Autodesk Inventor part; units mm, degrees
ref_plane "YZ Plane" through (0, 0, 0) normal (1, 0, 0) x (0, 1, 0)
ref_plane "XZ Plane" through (0, 0, 0) normal (0, 1, 0) x (-1, 0, 0)
ref_plane "XY Plane" through (0, 0, 0) normal (0, 0, 1) x (1, 0, 0)
sketch "Sketch1" plane through (0, 0, 0) normal (1, 0, 0) x (0, 1, 0)
  line L0 (12, -9) -> (2, -9)
  line L1 (2, -9) -> (2, 41)
  line L2 (2, 41) -> (7, 41)
  line L3 (7, 41) -> (7, 31)
  line L4 (7, 31) -> (12, 31)
  line L5 (12, 31) -> (12, -9)
  line L6 (2, 111) -> (12, 111)
  line L7 (12, 111) -> (12, 71)
  line L8 (12, 71) -> (7, 71)
  line L9 (7, 71) -> (7, 61)
  line L10 (7, 61) -> (2, 61)
  line L11 (2, 61) -> (2, 111)
  line L12 (7, 54.5) -> (7, 55)
  line L13 (7, 55) -> (62, 55)
  arc A0 (64, 57) -> (62, 55) centre (64, 55) ccw
  line L14 (64, 57) -> (65, 57)
  arc A1 (67, 55) -> (65, 57) centre (65, 55) ccw
  line L15 (67, 55) -> (102, 55)
  arc A2 (104, 57) -> (102, 55) centre (104, 55) ccw
  line L16 (104, 57) -> (105, 57)
  arc A3 (107, 55) -> (105, 57) centre (105, 55) ccw
  line L17 (107, 55) -> (107, 47)
  arc A4 (105, 45) -> (107, 47) centre (105, 47) ccw
  line L18 (105, 45) -> (104, 45)
  arc A5 (102, 47) -> (104, 45) centre (104, 47) ccw
  line L19 (102, 47) -> (67, 47)
  arc A6 (65, 45) -> (67, 47) centre (65, 47) ccw
  line L20 (65, 45) -> (64, 45)
  arc A7 (62, 47) -> (64, 45) centre (64, 47) ccw
  line L21 (62, 47) -> (7, 47)
  line L22 (7, 47) -> (7, 47.5)
  line L23 (7, 47.5) -> (-5, 47.5)
  line L24 (-5, 47.5) -> (-5, 41)
  line L25 (-5, 41) -> (0, 41)
  line L26 (0, 41) -> (0, 2.0396)
  line L27 (0, 2.0396) -> (0.3922, 1.9612)
  line L28 (0.3922, 1.9612) -> (0, 1.0198)
  line L29 (0, 1.0198) -> (0, 0)
  line L30 (0, 0) -> (-0.3922, 0.0784)
  line L31 (-0.3922, 0.0784) -> (-15.377, -35.885)
  line L32 (-15.377, -35.885) -> (-19.9924, -33.9619)
  line L33 (-19.9924, -33.9619) -> (-22.4924, -39.9619)
  line L34 (-22.4924, -39.9619) -> (-11.4155, -44.5773)
  line L35 (-11.4155, -44.5773) -> (-11.2232, -44.1158)
  line L36 (-11.2232, -44.1158) -> (39.5461, -65.2696)
  arc A8 (42.1615, -64.1927) -> (39.5461, -65.2696) centre (41.3922, -66.0388) ccw
  line L37 (42.1615, -64.1927) -> (43.0845, -64.5773)
  arc A9 (44.1615, -67.1927) -> (43.0845, -64.5773) centre (42.3153, -66.4235) ccw
  line L38 (44.1615, -67.1927) -> (76.4692, -80.6542)
  arc A10 (79.0845, -79.5773) -> (76.4692, -80.6542) centre (78.3153, -81.4235) ccw
  line L39 (79.0845, -79.5773) -> (80.0076, -79.9619)
  arc A11 (81.0845, -82.5773) -> (80.0076, -79.9619) centre (79.2384, -81.8081) ccw
  line L40 (81.0845, -82.5773) -> (78.0076, -89.9619)
  arc A12 (75.3922, -91.0388) -> (78.0076, -89.9619) centre (76.1615, -89.1927) ccw
  line L41 (75.3922, -91.0388) -> (74.4692, -90.6542)
  arc A13 (73.3922, -88.0388) -> (74.4692, -90.6542) centre (75.2384, -88.8081) ccw
  line L42 (73.3922, -88.0388) -> (41.0845, -74.5773)
  arc A14 (38.4692, -75.6542) -> (41.0845, -74.5773) centre (39.2384, -73.8081) ccw
  line L43 (38.4692, -75.6542) -> (37.5461, -75.2696)
  arc A15 (36.4692, -72.6542) -> (37.5461, -75.2696) centre (38.3153, -73.4235) ccw
  line L44 (36.4692, -72.6542) -> (-14.3001, -51.5004)
  line L45 (-14.3001, -51.5004) -> (-14.1078, -51.0388)
  line L46 (-14.1078, -51.0388) -> (-25.1847, -46.4235)
  line L47 (-25.1847, -46.4235) -> (-27.6847, -52.4235)
  line L48 (-27.6847, -52.4235) -> (-23.0693, -54.3465)
  line L49 (-23.0693, -54.3465) -> (-38.8385, -92.1927)
  line L50 (-38.8385, -92.1927) -> (-47.3001, -86.5004)
  line L51 (-47.3001, -86.5004) -> (-30.377, -45.885)
  line L52 (-30.377, -45.885) -> (-39.6078, -42.0388)
  line L53 (-39.6078, -42.0388) -> (-35.7616, -32.8081)
  line L54 (-35.7616, -32.8081) -> (-26.5308, -36.6542)
  line L55 (-26.5308, -36.6542) -> (-10, 3.0198)
  line L56 (-10, 3.0198) -> (-10, 46)
  line L57 (-10, 46) -> (-20, 46)
  line L58 (-20, 46) -> (-20, 56)
  line L59 (-20, 56) -> (-10, 56)
  line L60 (-10, 56) -> (-10, 100)
  line L61 (-10, 100) -> (0, 102)
  line L62 (0, 102) -> (0, 61)
  line L63 (0, 61) -> (-5, 61)
  line L64 (-5, 61) -> (-5, 54.5)
  line L65 (-5, 54.5) -> (7, 54.5)
  line L66 (0, 51) -> (107, 51)
  line L67 (79.5461, -86.2696) -> (-37.6847, -37.4235)
sketch "Sketch2" plane through (0, 0, 0) normal (1, 0, 0) x (0, 1, 0)
  line L0 (0, 0) -> (0, 51)
  line L1 (0, 51) -> (15, 51)
  line L2 (15, 51) -> (15, 101)
  line L3 (15, 101) -> (65, 101)
  line L4 (101.707, 46.9392) -> (84.707, 46.9392)
  line L5 (84.707, 46.9392) -> (34.707, 46.9392)
  line L6 (15, 51) -> (15, 60)
  line L7 (0, 0) -> (0, 1)
  line L8 (0, 1) -> (110.5886, -21.1178)
  line L9 (50.3822, 41.5) -> (30.3822, 41.5)
  line L10 (30.3822, 41.5) -> (30.3822, 0.5)
  line L11 (30.3822, 0.5) -> (50.3822, 0.5)
  line L12 (50.3822, 0.5) -> (50.3822, 41.5)
  line L13 (50.3822, 0.5) -> (45.3822, 0.5)
  line L14 (45.3822, 0.5) -> (45.3822, -3.5)
  line L15 (45.3822, -3.5) -> (35.3822, -3.5)
  circle A0 centre (45.3822, -3.5) radius 2
  circle A1 centre (35.3822, -3.5) radius 2
  line L16 (50.3822, 21) -> (30.3822, 21)
  circle A2 centre (45.3822, 45.5) radius 2
  circle A3 centre (35.3822, 45.5) radius 2
  line L17 (65, 101) -> (65, -12.0001)
  line L18 (0, 51) -> (107.1279, 51)
  line L19 (65, 51) -> (55, 51)
  line L20 (15, 51) -> (25, 51)
  line L21 (-5.3847, -50.9231) -> (-24.6156, -97.0769)
  line L22 (-24.6156, -97.0769) -> (21.5382, -116.3077)
  line L23 (21.5382, -116.3077) -> (65, -12.0001)
  line L24 (15, 51) -> (15, -19)
  line L25 (-5.3847, -50.9231) -> (7.9166, -19)
  line L26 (15, -19) -> (7.9166, -19)
  line L27 (30.9296, -55.7624) -> (12.468, -48.0701)
  line L28 (12.468, -48.0701) -> (28.2374, -10.224)
  line L29 (28.2374, -10.224) -> (46.6989, -17.9163)
  line L30 (46.6989, -17.9163) -> (30.9296, -55.7624)
  circle A4 centre (43.622, -12.3009) radius 2
  circle A5 centre (34.3912, -8.4548) radius 2
  circle A6 centre (24.7757, -57.5317) radius 2
  circle A7 centre (15.545, -53.6855) radius 2
  line L31 (65, 51) -> (65, 41)
  line L32 (65, 41) -> (63.5, 41)
  line L33 (63.5, 41) -> (63.5, 61)
  line L34 (63.5, 61) -> (65, 61)
  line L35 (65, 61) -> (65, 41)
  line L36 (63.5, 61) -> (57.5, 61)
  line L37 (57.5, 61) -> (56, 61)
  line L38 (56, 61) -> (56, 41)
  line L39 (56, 41) -> (57.5, 41)
  line L40 (57.5, 41) -> (57.5, 61)
  line L41 (65, 51) -> (60.5, 51)
  circle A8 centre (60.5, 51) radius 1.5
  line L42 (44.6152, -60.9232) -> (43.2306, -60.3463)
  line L43 (43.2306, -60.3463) -> (35.5383, -78.8078)
  line L44 (35.5383, -78.8078) -> (36.9229, -79.3847)
  line L45 (29.9998, -76.5001) -> (28.6152, -75.9231)
  line L46 (28.6152, -75.9231) -> (36.3076, -57.4616)
  line L47 (36.3076, -57.4616) -> (37.6922, -58.0386)
  line L48 (37.6922, -58.0386) -> (29.9998, -76.5001)
  circle A9 centre (36.6152, -68.4232) radius 1.5
  line L49 (-1.5387, -106.6923) -> (40, -7)
  line L50 (40, 101) -> (40, -7)
  line L51 (40, -68.0997) -> (40, -71.9997)
  circle A10 centre (-1.2309, -52.6538) radius 1.5
  line L52 (5.3845, -44.5769) -> (-2.3078, -63.0385)
  line L53 (-0.9232, -63.6154) -> (6.7691, -45.1539)
  line L54 (6.7691, -45.1539) -> (5.3845, -44.5769)
  line L55 (-2.3078, -63.0385) -> (-0.9232, -63.6154)
  line L56 (-0.1539, -42.2692) -> (-7.8463, -60.7308)
  line L57 (-7.8463, -60.7308) -> (-9.2309, -60.1538)
  line L58 (-1.5386, -41.6923) -> (-0.1539, -42.2692)
  line L59 (15, 41) -> (16.5, 41)
  line L60 (16.5, 41) -> (16.5, 61)
  line L61 (16.5, 61) -> (15, 61)
  line L62 (22.5, 61) -> (24, 61)
  line L63 (24, 61) -> (24, 41)
  line L64 (24, 41) -> (22.5, 41)
  line L65 (22.5, 41) -> (22.5, 61)
  circle A11 centre (19.5, 51) radius 1.5
  dimension "d0" = 51
  dimension "d1" = 15
  dimension "d2" = 50
  dimension "d3" = 50
  dimension "d11" = 17
  dimension "d12" = 50
  dimension "d23" = 9
  dimension "d34" = 1
  dimension "d35" = 78.69
  dimension "d36" = 20
  dimension "d37" = 41
  dimension "d38" = 5
  dimension "d39" = 4
  dimension "d40" = 10
  dimension "d41" = 4
  dimension "d42" = 4
  dimension "d43" = 10
  dimension "d47" = 10
  dimension "d48" = 70
  dimension "d86" = 10
  dimension "d87" = 1.5
  dimension "d88" = 20
  dimension "d89" = 6
  dimension "d90" = 1.5
  dimension "d91" = 20
  dimension "d92" = 4.5
  dimension "d93" = 3
extrude "Extrusion1" add sketch "Sketch2" along normal blind 1.5 contours L24 L59 L60 L18 A11 L65 L64 L63 L50 L9 L10 L11 L8 | L8 L49 L29 L28 L27 L22 L21 L57 L56 L58 L25 L26 L24 | L2 L61 L60 L18 | L18 L60 L59 L24 | L50 L15 A0 L14 L11 L12 L9 L5 A2 L38 L39 L40 L33 L32 L17 L8 | L8 L23 L42 L43 L44 L22 L49 L27 L30 L29 | L60 L61 L2 L3 L50 L18 L63 L62 L65 A11 | L50 L11 L14 A0 L15 | A11 L18 | L18 A11 | L32 L33 L5 L17 | L23 L51 L43 L42 | L58 L56 L57 L21 L25 | L5 L33 L18 L17 | L23 L44 L43 L51 | L3 L17 L34 L36 L37 L38 L18 L50 | L65 L62 L63 L18 | L18 L63 L64 L65 | L5 L40 L18 A8 L33 | L18 L33 L34 L17 | L18 L38 L5 A2 L50 | L40 L39 L38 L5 | L5 L38 L18 L40 | L18 A8 L40 L36 L33 | L18 L38 L37 L40 | A8 L18 | L18 A8 | L45 L46 L47 L48 | A9 | A10 | L54 L53 L55 L52
sketch "Sketch3" plane through (1.5, 0, 0) normal (1, 0, 0) x (0, 0, -1)
  line L0 (-101, 65) -> (-101, 15)
  line L1 (-101, 65) -> (-101, 55)
  line L2 (-101, 55) -> (-106, 55)
  line L3 (-106, 55) -> (-106, 35)
  line L4 (-106, 35) -> (-101, 35)
  line L5 (-101, 55) -> (-101, 50)
  line L6 (-101, 50) -> (-102.5, 50)
  line L7 (-102.5, 50) -> (-102.5, 40)
  line L8 (-102.5, 40) -> (-101, 40)
  line L9 (-101, 40) -> (-101, 50)
  line L10 (-1, 0) -> (21.1178, 110.5886)
  line L11 (116.3077, 21.5382) -> (97.0769, -24.6156)
  line L12 (112.4616, 12.3074) -> (117.0769, 10.3843)
  line L13 (117.0769, 10.3843) -> (109.3846, -8.0772)
  line L14 (109.3846, -8.0772) -> (104.7692, -6.1541)
  line L15 (110.5385, 7.692) -> (111.9231, 7.1151)
  line L16 (111.9231, 7.1151) -> (108.0769, -2.1156)
  line L17 (108.0769, -2.1156) -> (106.6923, -1.5387)
  point P0 (0, 0)
  point P1 (106.6923, -1.5387)
  dimension "d66" = 10
  dimension "d67" = 5
  dimension "d68" = 20
  dimension "d69" = 5
  dimension "d70" = 1.5
  dimension "d71" = 10
extrude "Extrusion2" add sketch "Sketch3" against normal blind 1.5 contours L0 L6 L7 L8 L4 L3 L2
extrude "Extrusion3" add sketch "Sketch3" against normal blind 1.5 contours L12 L13 L14 L11 L17 L16 L15
sketch "Sketch4" plane through (1.5, 0, 0) normal (1, 0, 0) x (0, 0, -1)
  line L0 (-101, 15) -> (19, 15)
  line L1 (-101, 15) -> (-101, 30)
  line L2 (-101, 35) -> (-101, 15)
  line L3 (-101, 30) -> (-81, 30)
  line L4 (-81, 30) -> (-61, 30)
  line L5 (-61, 30) -> (-61, 26)
  line L6 (-61, 26) -> (-81, 26)
  line L7 (-81, 26) -> (-81, 30)
  line L8 (-71, 30) -> (-71, 33)
  line L9 (-71, 33) -> (-71, 23)
  circle A0 centre (-71, 33) radius 1.5
  circle A1 centre (-71, 23) radius 1.5
  point P0 (0, 0)
  dimension "d76" = 15
  dimension "d77" = 20
  dimension "d78" = 20
  dimension "d79" = 4
  dimension "d80" = 3
  dimension "d81" = 10
  dimension "d82" = 3
  dimension "d83" = 3
extrude "Extrusion6" cut sketch "Sketch2" along normal blind 1.5 contours L2 L61 L60 L18 | L18 L60 L59 L24 | A11 L18 | L18 A11 | L32 L33 L5 L17 | L58 L56 L57 L21 L25 | L5 L33 L18 L17 | L65 L62 L63 L18 | L18 L63 L64 L65 | L18 L33 L34 L17 | L40 L39 L38 L5 | L5 L38 L18 L40 | L18 L38 L37 L40 | A8 L18 | L18 A8 | A10 | L54 L53 L55 L52
extrude "Extrusion7" cut sketch "Sketch2" along normal blind 1.5 contours L23 L51 L43 L42 | L23 L44 L43 L51 | L45 L46 L47 L48 | A9
extrude "Extrusion8" cut sketch "Sketch4" against normal blind 1.5 contours A0 | L4 L9 L6 L7 | L4 L5 L6 L9
extrude "Extrusion9" cut sketch "Sketch4" against normal blind 10 contours A1
properties part number "centralFinal"
Check sheet for the modelled part. Datum: model origin and axes. Units: mm. A direction names the side the tool comes from. Coordinates: 2 decimals unless noted, no trailing zeros. Loops run counter-clockwise (first coordinate to the right, second up) from the corner with the lowest first, then second, coordinate; pieces in that order, holes last. Notation, with made-up numbers: M 77,0 L 121,0 A21 ccw 121,24 Z; hole C -9,-11.75 d11. An arc over 180 degrees is marked long. Answer as a JSON object with one key per item and string values.
1. Sectioned sample at A-A on z = -3.5. Record the cut outline in (x, y).
Outcome:
{"outline": "M 0,15 L 1.5,15 L 1.5,33.38 L 0,33.38 Z; M 0,37.38 L 1.5,37.38 L 1.5,43.38 L 0,43.38 Z; M 0,47.38 L 1.5,47.38 L 1.5,65 L 0,65 Z"}
2. Access from +Z, -Z, +X, -X, +Y, -Y to the whole of each face (thin tool, end or side, straight path). Record for faces 1 (the flat face through (0.76, 1.283, -113.285)), 2 (the flat face through (0.7, 37.3, -14)).
Outcome:
{"face 1": "-Z, +X, -X, -Y", "face 2": "+X, -X"}
3. Sectioned sample at D-D on z = 88. Record the cut outline in (x, y).
Outcome:
{"outline": "M 0,15 L 1.5,15 L 1.5,65 L 0,65 Z"}
4. Depth check by flat-ended pin: P1, Ø5, axis at y = 36.62, z = -68.42, coming from the +X side. Enter the tip coordinate at first touch or a pass-through.
Outcome:
{"P1": "x = 1.5"}
5. Release check for a two-part mould opening along Z. For faces 3 (the cylindrical face through (0.74, 26.623, -56.766)), 4 (the flat face through (0.74, 54.665, -36.804)), 5 (the flat face through (0.74, 3.12, -30.51)) record: pulls with the +Z half, pulls with the -Z half, needs draft (parallel to the pull), parting line crosses it, or undercut.
Outcome:
{"face 3": "undercut", "face 4": "pulls with the -Z half", "face 5": "pulls with the +Z half"}
6. Sectioned sample at C-C on z = -28. Record the cut outline in (x, y), and give its area (4 significant figures).
Outcome:
{"outline": "M 0,4.17 L 1.5,4.17 L 1.5,20.83 L 0,20.83 Z; M 0,42.5 L 1.5,42.5 L 1.5,58.33 L 0,58.33 Z", "area": "48.75 mm²"}
7. Sectioned sample at B-B on z = 45.5. Record the cut outline in (x, y), and give its area (3 significant figures).
Outcome:
{"outline": "M 0,16.5 L 1.5,16.5 L 1.5,22.5 L 0,22.5 Z; M 0,24 L 1.5,24 L 1.5,33.38 L 0,33.38 Z; M 0,37.38 L 1.5,37.38 L 1.5,43.38 L 0,43.38 Z; M 0,47.38 L 1.5,47.38 L 1.5,56 L 0,56 Z; M 0,57.5 L 1.5,57.5 L 1.5,63.5 L 0,63.5 Z", "area": "54.0 mm²"}
8. Scan lines: L1, parallel to Z at x = 0.4, y = 40.5; L2, parallel to Z at x = 1, y = 41; L3, parallel to Z at x = 1.25, y = 33. Record each from-to range of solid material in increasing order. Write a range as from..to.
Outcome:
{"L1": "-66.9..-32.79, -15.33..0.5, 41.5..101, 102.5..106", "L2": "-65.7..-31.59, -15.54..0.5, 41.5..101, 102.5..106", "L3": "-88.8..-69.3, -65.4..-50.79, -12.21..-9.89, -7.02..0.5, 41.5..69.5, 72.5..101"}
